Answer from the drawing. Dimensions are ordinates in mm from the lowest x, y and z of the part. A direction names the side the tool comes from. Coordinates: 2 decimals unless noted, no trailing zeros. Write each loop counter-clockwise with the first axis right and the second up, starting at its lowest first coordinate (ties: lowest second). Pieces come first, ordered by that corner, then holes. Notation, with made-up numbers: (60, 41.5) - (111, 41.5) arc R13 cw to (111, 58.5) - close; hole circle Ø4 at (13.25, 80.5). An arc over 180 degrees is marked (long way). Return JSON: item names as keys, results as strings.
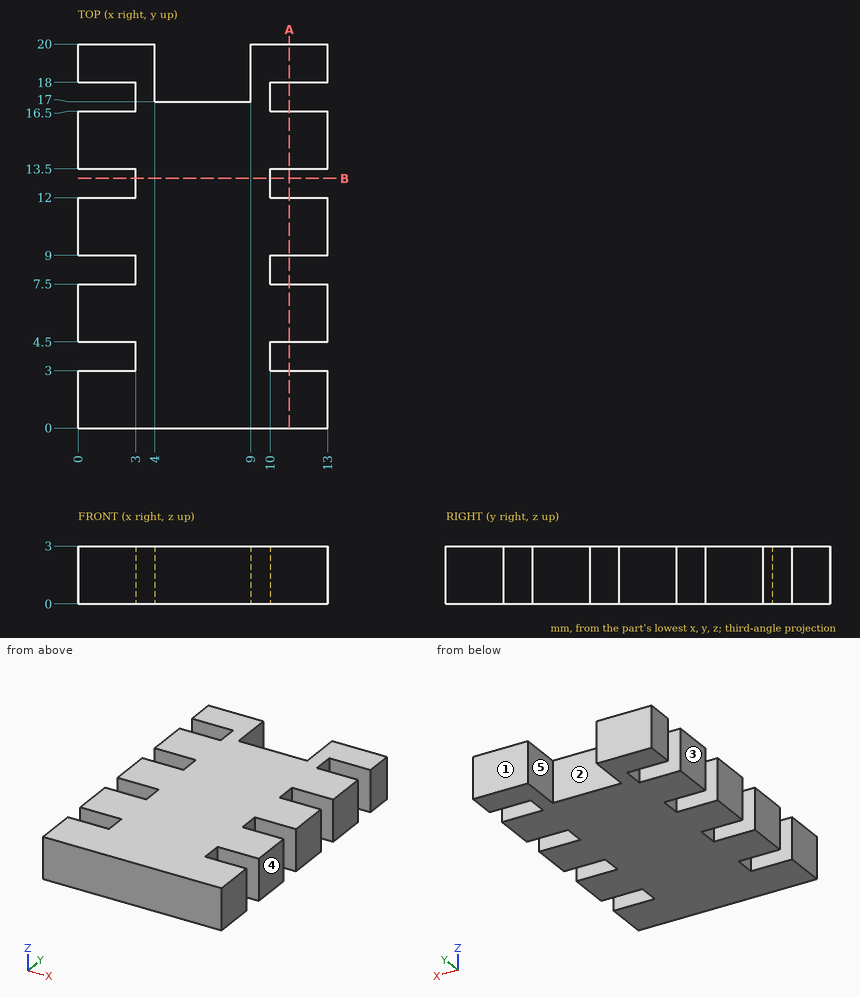
(1) Straight lines are drawn through the part: line 1 (Y direction, x = 11.25, z = 1.45); line 2 (Y direction, x = 4.5, z = 1.6); line 3 (X direction, y = 3.75, z = 0.65). For each, find the intervals that lie inside material, in ascending order. Write a range as from..to.
Answer:
{"line 1": "0..3, 4.5..7.5, 9..12, 13.5..16.5, 18..20", "line 2": "0..17", "line 3": "3..10"}
(2) Determine the mould class of the marked faces 1, 2 and 3 for opening direction X: +X half, -X half, draft (parallel to the pull), parting line (faces both ways), or undercut.
Answer:
{"face 1": "draft", "face 2": "undercut", "face 3": "-X half"}
(3) A cutting plane is placed at A-A (x = 11). Determine the outline of the cut face in (y, z).
Answer:
{"outline": "(0, 0) - (3, 0) - (3, 3) - (0, 3) - close; (4.5, 0) - (7.5, 0) - (7.5, 3) - (4.5, 3) - close; (9, 0) - (12, 0) - (12, 3) - (9, 3) - close; (13.5, 0) - (16.5, 0) - (16.5, 3) - (13.5, 3) - close; (18, 0) - (20, 0) - (20, 3) - (18, 3) - close"}
(4) A cutting plane is placed at B-B (y = 13). Determine the outline of the cut face in (x, z), and give its area (3 significant figures).
Answer:
{"outline": "(3, 0) - (10, 0) - (10, 3) - (3, 3) - close", "area": "21.0 mm²"}
(5) Which of the six approach directions +Z, -Z, +X, -X, +Y, -Y give full straight-line access (tool end or side, diameter ignored) to the marked faces 4 and 5?
Answer:
{"face 4": "+Z, -Z, +X, +Y, -Y", "face 5": "+Z, -Z, +Y"}
